Autodesk Inventor part; units mm, degrees
ref_plane "Work Plane1" through (0, 0, 0) normal (0, 0, 1) x (1, 0, 0)
ref_plane "Work Plane2" through (-150.1545, -254.8124, 77.677) normal (0, 0, -1) x (0, 1, 0)
ref_plane "YZ Plane" through (0, 0, 0) normal (1, 0, 0) x (0, 1, 0)
ref_plane "Work Plane1" through (0, 0, 0) normal (0, 0, 1) x (1, 0, 0)
sketch "Sketch1" plane through (0, 0, 0) normal (0, 0, 1) x (1, 0, 0)
  circle A0 centre (-5.3931, -215.9272) radius 1.778 construction
  line L0 (0.9569, -209.5772) -> (-11.7431, -209.5772)
  line L1 (-11.7431, -209.5772) -> (-11.7431, -222.2772)
  line L2 (-11.7431, -222.2772) -> (0.9569, -222.2772)
  line L3 (0.9569, -222.2772) -> (0.9569, -209.5772)
  line L4 (0.9569, -209.5772) -> (-11.7431, -222.2772) construction
  line L5 (-11.7431, -209.5772) -> (0.9569, -222.2772) construction
  circle A1 centre (-5.3931, -215.9272) radius 1.7
  point P0 (0, 0)
  dimension "d0" = 12.7
  dimension "d1" = 12.7
  dimension "d2" = 3.4
ref_plane "Work Plane2" through (-150.1545, -254.8124, 77.677) normal (0, 0, -1) x (0, 1, 0)
extrude "Extrusion1" add sketch "Sketch1" along normal up to surface (77.677 mm away)
ref_plane "Work Plane3" through (0, 0, 9) normal (0, 0, -1) x (-1, 0, 0)
sketch "Sketch2" plane through (0, 0, 9) normal (0, 0, -1) x (-1, 0, 0)
  circle A0 centre (5.3931, -215.9272) radius 1.7 construction
  circle A1 centre (5.3931, -215.9272) radius 3.45 construction
  line L0 (11.7431, -218.915) -> (3.6681, -218.915)
  line L1 (3.6681, -218.915) -> (1.9431, -215.9272)
  line L2 (1.9431, -215.9272) -> (3.6681, -212.9394)
  line L3 (3.6681, -212.9394) -> (11.7431, -212.9394)
  line L4 (11.7431, -212.9394) -> (11.7431, -218.915)
  line L5 (11.7431, -209.5772) -> (11.7431, -222.2772)
  line L6 (11.7431, -218.915) -> (3.6681, -218.915)
  line L7 (3.6681, -218.915) -> (1.9431, -215.9272)
  line L8 (1.9431, -215.9272) -> (3.6681, -212.9394)
  line L9 (3.6681, -212.9394) -> (11.7431, -212.9394)
  line L10 (11.7431, -212.9394) -> (11.7431, -218.915)
  point P0 (0, 0)
  dimension "d6" = 6.9
extrude "Extrusion2" cut sketch "Sketch2" against normal blind 4.4
ref_plane "Work Plane4" through (-11.7431, -222.2772, 68.677) normal (0, 0, 1) x (1, 0, 0)
sketch "Sketch3" plane through (-11.7431, -222.2772, 68.677) normal (0, 0, 1) x (1, 0, 0)
  line L0 (0, 9.3378) -> (8.075, 9.3378)
  line L1 (8.075, 9.3378) -> (9.8, 6.35)
  line L2 (9.8, 6.35) -> (8.075, 3.3622)
  line L3 (8.075, 3.3622) -> (0, 3.3622)
  line L4 (0, 3.3622) -> (0, 9.3378)
  circle A0 centre (6.35, 6.35) radius 1.7 construction
  circle A1 centre (6.35, 6.35) radius 3.45 construction
  point P0 (11.7431, 222.2772)
  dimension "d10" = 6.9
extrude "Extrusion3" cut sketch "Sketch3" against normal blind 4.4
properties part number "supports"
Can you work these out from the model? Positions are in its coordinate system, mm. A direction names the side the tool comes from. Give positions to 0.01 mm unless a question says otherwise; leave off trailing zeros. Loops run counter-clockwise (first coordinate to the right, second up) from the corner with the lowest first, then second, coordinate; pieces in that order, holes last. Notation, with made-up numbers: (45.25, 18.25) -> (92.25, 18.25) arc R13 ccw to (92.25, 40.25) -> close; hole circle Ø5 at (-0.75, 58.5). An arc over 180 degrees is marked (long way). Return JSON: item names as keys, results as strings.
Q1. I want a section at A-A, the plane x = -10. List the corners of the cut face in (y, z) for me (3 decimals), then the cut area to 3 significant figures.
Checks:
{"outline": "(-222.277, 0) -> (-209.577, 0) -> (-209.577, 77.677) -> (-222.277, 77.677) -> close; hole (-218.915, 9) -> (-212.939, 9) -> (-212.939, 13.4) -> (-218.915, 13.4) -> close; hole (-218.915, 64.277) -> (-212.939, 64.277) -> (-212.939, 68.677) -> (-218.915, 68.677) -> close", "area": "934 mm2"}
Q2. I need wall thicknesses on probe 1 along Z at (x, y) = (-10, -214); probe 2 along Y at (x, z) = (-5.5, 25); probe 3 along X at (y, z) = (-215.25, 20). Which ranges of each line are inside material? Lowest first, please.
Checks:
{"probe 1": "z = 0 to 9, 13.4 to 64.28, 68.68 to 77.68", "probe 2": "y = -222.28 to -217.62, -214.23 to -209.58", "probe 3": "x = -11.74 to -6.95, -3.83 to 0.96"}
Q3. On a 3-axis mill with a long thin cutter (end or side, diameter ignored), from which of +Z, -Z, +X, -X, +Y, -Y can I reach the whole of each face in a straight line? I mean faces 1 (the face through (-8, -216, 13.4)), 2 (the face through (0.957, -216, 38)). Say none if no direction works.
Checks:
{"face 1": "-X", "face 2": "+Z, -Z, +X, +Y, -Y"}
Q4. I want a section at B-B, the plane z = 43.5. List the corners of the cut face in (x, y) for me.
Checks:
{"outline": "(-11.74, -222.28) -> (0.96, -222.28) -> (0.96, -209.58) -> (-11.74, -209.58) -> close; hole circle Ø3.4 at (-5.39, -215.93)"}
Q5. We'd pull the mould along X, two halves only. Please class faces 3 (the face through (-5.762, -214.268, 73.114)), 4 (the face through (-2.794, -214.454, 11.169)), 5 (the face through (-8, -216, 9)): released by +X, released by -X, zero draft, split by the parting line, or undercut.
Checks:
{"face 3": "undercut", "face 4": "released by -X", "face 5": "zero draft"}
Q6. I want a section at D-D, the plane x = -2.75. List the corners of the cut face in (y, z) for me.
Checks:
{"outline": "(-222.28, 0) -> (-209.58, 0) -> (-209.58, 77.68) -> (-222.28, 77.68) -> close; hole (-217.32, 9) -> (-214.53, 9) -> (-214.53, 13.4) -> (-217.32, 13.4) -> close; hole (-217.32, 64.28) -> (-214.53, 64.28) -> (-214.53, 68.68) -> (-217.32, 68.68) -> close"}
Q7. I want a section at C-C, the plane z = 65. List the corners of the cut face in (x, y) for me (3 decimals).
Checks:
{"outline": "(-11.743, -222.277) -> (0.957, -222.277) -> (0.957, -209.577) -> (-11.743, -209.577) -> (-11.743, -212.939) -> (-3.668, -212.939) -> (-1.943, -215.927) -> (-3.668, -218.915) -> (-11.743, -218.915) -> close"}
